from build123d import *

# Parameters (mm, degrees)
SKETCH1_W           = 100
SKETCH1_H           = 290
BOSS_EXTRUDE1_DEPTH = 6
SKETCH2_W           = 62
SKETCH2_H           = 26
CUT_EXTRUDE1_DEPTH  = 7
SKETCH3_W           = 52
SKETCH3_H           = 290
CUT_EXTRUDE2_DEPTH  = 2
SKETCH4_R           = 2.5
SKETCH4_R_2         = 5.25
SKETCH4_R_3         = 3.3
SKETCH4_R_4         = 2.1
CUT_EXTRUDE4_DEPTH  = 21
FILLET1_R           = 3
FILLET2_R           = 6
CHAMFER1_SIZE       = 2
SKETCH5_R           = 5.75
CUT_EXTRUDE5_DEPTH  = 5
CHAMFER2_SIZE       = 2


with BuildPart() as part:
    # Sketch1 → Boss-Extrude1 (new, symmetric)
    with BuildSketch(Plane.XY):
        Rectangle(SKETCH1_W, SKETCH1_H)
    extrude(amount=BOSS_EXTRUDE1_DEPTH, both=True)

    # Sketch2 → Cut-Extrude1 (cut)
    with BuildSketch(Plane.XY.offset(6)):
        with Locations((0, 132)):
            Rectangle(SKETCH2_W, SKETCH2_H)
    extrude(amount=-CUT_EXTRUDE1_DEPTH, mode=Mode.SUBTRACT)

    # Sketch3 → Cut-Extrude2 (cut)
    with BuildSketch(Plane.XY.offset(6)):
        Rectangle(SKETCH3_W, SKETCH3_H)
    extrude(amount=-CUT_EXTRUDE2_DEPTH, mode=Mode.SUBTRACT)

    # Sketch4 → Cut-Extrude4 (cut)
    with BuildSketch(Plane.XY.offset(-6)):
        with Locations((-23, 139)):
            Circle(SKETCH4_R)
        with Locations((23, 139)):
            Circle(SKETCH4_R)
        with Locations((23, 126)):
            Circle(SKETCH4_R)
        with Locations((-23, 126)):
            Circle(SKETCH4_R)
        with Locations(Location((0, 34, 0), (0, 0, 180))):
            Circle(SKETCH4_R_2)
        with Locations(Location((-18, 59, 0), (0, 0, 180))):
            Circle(SKETCH4_R_3)
        with Locations(Location((-18, 34, 0), (0, 0, 180))):
            Circle(SKETCH4_R_3)
        with Locations(Location((-18, 11.5, 0), (0, 0, 180))):
            Circle(SKETCH4_R_3)
        with Locations((-36, 81.25)):
            Circle(SKETCH4_R_4)
        with Locations((-36, 70)):
            Circle(SKETCH4_R_4)
        with Locations((-36, 58.75)):
            Circle(SKETCH4_R_4)
        with Locations((-36, 10)):
            Circle(SKETCH4_R_4)
        with Locations((-36, -110)):
            Circle(SKETCH4_R_4)
        with Locations((-36, -50)):
            Circle(SKETCH4_R_4)
        with Locations(Location((-18, -102.5, 0), (0, 0, 180))):
            Circle(SKETCH4_R_3)
        with Locations(Location((-18, -125, 0), (0, 0, 180))):
            Circle(SKETCH4_R_3)
        with Locations(Location((18, -102.5, 0), (0, 0, 180))):
            Circle(SKETCH4_R_3)
        with Locations(Location((18, -125, 0), (0, 0, 180))):
            Circle(SKETCH4_R_3)
        with Locations(Location((0, -132.5, 0), (0, 0, 180))):
            Circle(SKETCH4_R_3)
        with Locations(Location((36, 81.25, 0), (0, 0, 180))):
            Circle(SKETCH4_R_4)
        with Locations(Location((36, 70, 0), (0, 0, 180))):
            Circle(SKETCH4_R_4)
        with Locations(Location((36, 58.75, 0), (0, 0, 180))):
            Circle(SKETCH4_R_4)
        with Locations(Location((18, 59, 0), (0, 0, 180))):
            Circle(SKETCH4_R_3)
        with Locations(Location((18, 11.5, 0), (0, 0, 180))):
            Circle(SKETCH4_R_3)
        with Locations(Location((18, 34, 0), (0, 0, 180))):
            Circle(SKETCH4_R_3)
        with Locations(Location((36, 10, 0), (0, 0, 180))):
            Circle(SKETCH4_R_4)
        with Locations(Location((36, -50, 0), (0, 0, 180))):
            Circle(SKETCH4_R_4)
        with Locations(Location((36, -110, 0), (0, 0, 180))):
            Circle(SKETCH4_R_4)
    extrude(amount=CUT_EXTRUDE4_DEPTH, mode=Mode.SUBTRACT)

    # Fillet1
    fillet1_edges = [part.edges().sort_by_distance(p)[0] for p in [
        (-31, 119, 2.5),
        (31, 119, 2.5),
    ]]
    fillet(fillet1_edges, radius=FILLET1_R)

    # Fillet2
    fillet2_edges = [part.edges().sort_by_distance(p)[0] for p in [
        (-50, 145, 0),
        (50, 145, 0),
        (50, -145, 0),
        (-50, -145, 0),
    ]]
    fillet(fillet2_edges, radius=FILLET2_R)

    # Chamfer1
    chamfer1_edges = [part.edges().sort_by_distance(p)[0] for p in [
        (35, -145, 6),
        (48.242640687, -143.242640687, 6),
        (50, 0, 6),
        (48.242640687, 143.242640687, 6),
        (37.5, 145, 6),
        (-35, -145, 6),
        (-48.242640687, -143.242640687, 6),
        (-50, 0, 6),
        (-48.242640687, 143.242640687, 6),
        (-37.5, 145, 6),
    ]]
    chamfer(chamfer1_edges, length=CHAMFER1_SIZE)

    # Sketch5 → Cut-Extrude5 (cut)
    with BuildSketch(Plane.XY.offset(4)):
        with Locations((-18, 59)):
            Circle(SKETCH5_R)
        with Locations((-18, 34)):
            Circle(SKETCH5_R)
        with Locations((-18, 11.5)):
            Circle(SKETCH5_R)
        with Locations((18, 11.5)):
            Circle(SKETCH5_R)
        with Locations((18, 34)):
            Circle(SKETCH5_R)
        with Locations((18, 59)):
            Circle(SKETCH5_R)
        with Locations((18, -102.5)):
            Circle(SKETCH5_R)
        with Locations((-18, -102.5)):
            Circle(SKETCH5_R)
        with Locations((-18, -125)):
            Circle(SKETCH5_R)
        with Locations((0, -132.5)):
            Circle(SKETCH5_R)
        with Locations((18, -125)):
            Circle(SKETCH5_R)
    extrude(amount=-CUT_EXTRUDE5_DEPTH, mode=Mode.SUBTRACT)

    # Chamfer2
    chamfer2_edges = [part.edges().sort_by_distance(p)[0] for p in [
        (5.25, 34, 4),
    ]]
    chamfer(chamfer2_edges, length=CHAMFER2_SIZE)


solid = part.part
Can you work these out from the model? Positions are in its coordinate system, mm. A direction names the side the tool comes from. Coordinates: 2 decimals unless noted, no trailing zeros. Order: outer loops, then holes, each group sorted by start corner. A loop starts at its lowest first (then second) coordinate and runs counter-clockwise, first axis right, second up. Notation, with made-up numbers: (81.5, -38.75) - (130.5, -38.75) arc R15 ccw to (130.5, -13.75) - close; hole circle Ø10 at (43.5, 1.25). An arc over 180 degrees is marked (long way). Answer as a JSON object with one key per item and string values. Group by question number.
Q1. On a 3-axis mill with a long thin cutter (end or side, diameter ignored), from which of +Z, -Z, +X, -X, +Y, -Y can I reach the whole of each face in a straight line? I mean faces 4 (the face through (16.754, 28.387, 1.535)), 5 (the face through (-2.82, 29.57, -2.06)), 6 (the face through (31, 133, 3)). Say none if no direction works.
Q2. Imagine slicing it at C-C (y = 23.5). Please give me the cut outline in (x, z).
Q3. I need wall thicknesses on line 1 (X direction, y = -125, z = -2.15); line 2 (Y direction, x = -18, z = 0.65); line 3 (X direction, y = 81.25, z = 1.75). Which ranges of each line are inside material? Lowest first, please. Write a range as from..to.
Q4. Imagine slicing it at B-B (y = 126). Please give me the cut outline in (x, z).
Q5. Imagine slicing it at A-A (x = 0). Please give me the cut outline in (y, z), and give its area (3 significant figures).
Q6. Will these pins go through, and if not, where does the flat tip stop? P1, Ø10.5, axis at x = -18, y = -102.5, coming from the +Z side; P2, Ø8, axis at x = -18.5, y = 8.5, coming from the -Z side; P3, Ø1, axis at y = -75, z = 5, coming from the -X side; P4, Ø3, axis at x = 10.5, y = -71, coming from the +Z side.
Q7. We'd pull the mould along X, two halves only. Please class faces 1 (the face through (-37, 2, 6)), 2 (the face through (-1.246, -138.113, 1.535)), 3 (the face through (47.331, -142.405, 5.236)): +X half, -X half, draft (parallel to the pull), parting line (faces both ways), or undercut.
Determined:
{
 "1": {"face 4": "+Z", "face 5": "+Z, -Z", "face 6": "+Z, +Y"},
 "2": {"outline": "(-50, -6) - (50, -6) - (50, 4) - (48, 6) - (26, 6) - (26, 4) - (-26, 4) - (-26, 6) - (-48, 6) - (-50, 4) - close"},
 "3": {"line 1": "x = -50..-21.3, -14.7..14.7, 21.3..50", "line 2": "y = -145..-130.75, -119.25..-108.25, -96.75..5.75, 17.25..28.25, 39.75..53.25, 64.75..119", "line 3": "x = -50..-38.1, -33.9..33.9, 38.1..50"},
 "4": {"outline": "(-50, -6) - (-25.5, -6) - (-25.5, -1) - (-31, -1) - (-31, 6) - (-48, 6) - (-50, 4) - close; (-20.5, -6) - (20.5, -6) - (20.5, -1) - (-20.5, -1) - close; (25.5, -6) - (50, -6) - (50, 4) - (48, 6) - (31, 6) - (31, -1) - (25.5, -1) - close"},
 "5": {"outline": "(-145, -6) - (-135.8, -6) - (-135.8, -1) - (-138.25, -1) - (-138.25, 4) - (-145, 4) - close; (-129.2, -6) - (28.75, -6) - (28.75, 2) - (26.75, 4) - (-126.75, 4) - (-126.75, -1) - (-129.2, -1) - close; (39.25, -6) - (145, -6) - (145, -1) - (119, -1) - (119, 4) - (41.25, 4) - (39.25, 2) - close", "area": "2,570 mm2"},
 "6": {"P1": "stops at z = -1", "P2": "stops at z = -6", "P3": "stops at x = -49.5", "P4": "stops at z = 4"},
 "7": {"face 1": "draft", "face 2": "undercut", "face 3": "+X half"}
}
